Here's how the part is built. I have some questions about the finished solid (model axes, mm). Round coordinates to 2 decimals unless told otherwise and drop trailing zeros. Loops run counter-clockwise (first coordinate to the right, second up) from the corner with the lowest first, then second, coordinate; pieces in that order, holes last. Notation, with made-up numbers: M 53.25,-26.75 L 62.25,-26.75 A24 cw 62.25,-2.75 Z; hole C 18.25,11 d9. An arc over 180 degrees is marked long. Answer as a JSON object with one key per item and string values.
from build123d import *

# Parameters (mm, degrees)
SKETCH1_R           = 88.9
BOSS_EXTRUDE1_DEPTH = 6.35
CUT_EXTRUDE1_REACH  = 8.35
SKETCH2_R           = 1
CUT_EXTRUDE2_REACH  = 8.35
SKETCH4_R           = 1.5875


with BuildPart() as part:
    # Sketch1 → Boss-Extrude1 (new body)
    with BuildSketch(Plane(origin=(0, 0, 0), x_dir=(1, 0, 0), z_dir=(0, 1, 0))):
        Circle(SKETCH1_R)
    extrude(amount=BOSS_EXTRUDE1_DEPTH)

    # Sketch2 → Cut-Extrude1 (cut, up to next)
    with BuildSketch(Plane.XZ, mode=Mode.PRIVATE) as cut_extrude1_sk1:
        with Locations((2.411677935, -76.2)):
            Circle(SKETCH2_R)
    cut_extrude1_tool1 = extrude(cut_extrude1_sk1.sketch, amount=-CUT_EXTRUDE1_REACH, mode=Mode.PRIVATE) & part.part
    add(cut_extrude1_tool1.solids().sort_by_distance((2.411678, 0, -76.2))[0], mode=Mode.SUBTRACT)
    # Sketch2 → Cut-Extrude1 (cut, up to next)
    with BuildSketch(Plane.XZ, mode=Mode.PRIVATE) as cut_extrude1_sk2:
        with Locations((-2.425285476, -76.2)):
            Circle(SKETCH2_R)
    cut_extrude1_tool2 = extrude(cut_extrude1_sk2.sketch, amount=-CUT_EXTRUDE1_REACH, mode=Mode.PRIVATE) & part.part
    add(cut_extrude1_tool2.solids().sort_by_distance((-2.425285, 0, -76.2))[0], mode=Mode.SUBTRACT)
    # Sketch2 → Cut-Extrude1 (cut, up to next)
    with BuildSketch(Plane.XZ, mode=Mode.PRIVATE) as cut_extrude1_sk3:
        with Locations((-76.2, -2.411677935)):
            Circle(SKETCH2_R)
    cut_extrude1_tool3 = extrude(cut_extrude1_sk3.sketch, amount=-CUT_EXTRUDE1_REACH, mode=Mode.PRIVATE) & part.part
    add(cut_extrude1_tool3.solids().sort_by_distance((-76.2, 0, -2.411678))[0], mode=Mode.SUBTRACT)
    # Sketch2 → Cut-Extrude1 (cut, up to next)
    with BuildSketch(Plane.XZ, mode=Mode.PRIVATE) as cut_extrude1_sk4:
        with Locations((-76.2, 2.425285476)):
            Circle(SKETCH2_R)
    cut_extrude1_tool4 = extrude(cut_extrude1_sk4.sketch, amount=-CUT_EXTRUDE1_REACH, mode=Mode.PRIVATE) & part.part
    add(cut_extrude1_tool4.solids().sort_by_distance((-76.2, 0, 2.425285))[0], mode=Mode.SUBTRACT)
    # Sketch2 → Cut-Extrude1 (cut, up to next)
    with BuildSketch(Plane.XZ, mode=Mode.PRIVATE) as cut_extrude1_sk5:
        with Locations((-2.411677935, 76.2)):
            Circle(SKETCH2_R)
    cut_extrude1_tool5 = extrude(cut_extrude1_sk5.sketch, amount=-CUT_EXTRUDE1_REACH, mode=Mode.PRIVATE) & part.part
    add(cut_extrude1_tool5.solids().sort_by_distance((-2.411678, 0, 76.2))[0], mode=Mode.SUBTRACT)
    # Sketch2 → Cut-Extrude1 (cut, up to next)
    with BuildSketch(Plane.XZ, mode=Mode.PRIVATE) as cut_extrude1_sk6:
        with Locations((2.425285476, 76.2)):
            Circle(SKETCH2_R)
    cut_extrude1_tool6 = extrude(cut_extrude1_sk6.sketch, amount=-CUT_EXTRUDE1_REACH, mode=Mode.PRIVATE) & part.part
    add(cut_extrude1_tool6.solids().sort_by_distance((2.425285, 0, 76.2))[0], mode=Mode.SUBTRACT)
    # Sketch2 → Cut-Extrude1 (cut, up to next)
    with BuildSketch(Plane.XZ, mode=Mode.PRIVATE) as cut_extrude1_sk7:
        with Locations((76.2, 2.411677935)):
            Circle(SKETCH2_R)
    cut_extrude1_tool7 = extrude(cut_extrude1_sk7.sketch, amount=-CUT_EXTRUDE1_REACH, mode=Mode.PRIVATE) & part.part
    add(cut_extrude1_tool7.solids().sort_by_distance((76.2, 0, 2.411678))[0], mode=Mode.SUBTRACT)
    # Sketch2 → Cut-Extrude1 (cut, up to next)
    with BuildSketch(Plane.XZ, mode=Mode.PRIVATE) as cut_extrude1_sk8:
        with Locations((76.2, -2.425285476)):
            Circle(SKETCH2_R)
    cut_extrude1_tool8 = extrude(cut_extrude1_sk8.sketch, amount=-CUT_EXTRUDE1_REACH, mode=Mode.PRIVATE) & part.part
    add(cut_extrude1_tool8.solids().sort_by_distance((76.2, 0, -2.425285))[0], mode=Mode.SUBTRACT)

    # Sketch4 → Cut-Extrude2 (cut, up to next)
    with BuildSketch(Plane.XZ, mode=Mode.PRIVATE) as cut_extrude2_sk1:
        with Locations((4.766839139, -13.885779707)):
            Circle(SKETCH4_R)
    cut_extrude2_tool1 = extrude(cut_extrude2_sk1.sketch, amount=-CUT_EXTRUDE2_REACH, mode=Mode.PRIVATE) & part.part
    add(cut_extrude2_tool1.solids().sort_by_distance((4.766839, 0, -13.88578))[0], mode=Mode.SUBTRACT)
    # Sketch4 → Cut-Extrude2 (cut, up to next)
    with BuildSketch(Plane.XZ, mode=Mode.PRIVATE) as cut_extrude2_sk2:
        with Locations((-14.408857547, 2.814686063)):
            Circle(SKETCH4_R)
    cut_extrude2_tool2 = extrude(cut_extrude2_sk2.sketch, amount=-CUT_EXTRUDE2_REACH, mode=Mode.PRIVATE) & part.part
    add(cut_extrude2_tool2.solids().sort_by_distance((-14.408858, 0, 2.814686))[0], mode=Mode.SUBTRACT)
    # Sketch4 → Cut-Extrude2 (cut, up to next)
    with BuildSketch(Plane.XZ, mode=Mode.PRIVATE) as cut_extrude2_sk3:
        with Locations((9.642018407, 11.071093644)):
            Circle(SKETCH4_R)
    cut_extrude2_tool3 = extrude(cut_extrude2_sk3.sketch, amount=-CUT_EXTRUDE2_REACH, mode=Mode.PRIVATE) & part.part
    add(cut_extrude2_tool3.solids().sort_by_distance((9.642018, 0, 11.071094))[0], mode=Mode.SUBTRACT)


solid = part.part
Item 1: I'm going to push flat-ended pins straight in: pin 1 Ø2.5 at (x, z) = (76.2, 2.41) entering from +Y; pin 2 Ø1.2 at (x, z) = (-76.2, -2.41) entering from +Y; pin 3 Ø1 at (y, z) = (4, -67) entering from +X; pin 4 Ø2 at (y, z) = (2.5, 8) entering from +X. Where does each tip first touch, or does it pass through?
Resolved:
{"pin 1": "y = 6.35", "pin 2": "through", "pin 3": "x = 59", "pin 4": "x = 88.62"}
Item 2: I want a section at A-A, the plane y = 1.5. State how many separate pieces and enclosed holes the cut face has, then the cut area to 3 significant figures.
Resolved:
{"separate pieces": "1", "enclosed holes": "11", "area": "24,800 mm²"}
Item 3: Please list where these lines run through material, in increasing order: probe 1 along Z at (x, y) = (2, 4.75); probe 2 along X at (y, z) = (3.5, 75.5); probe 3 along X at (y, z) = (2.75, -76.2). Write a range as from..to.
Resolved:
{"probe 1": "-88.88..-77.11, -75.29..75.29, 77.11..88.88", "probe 2": "-46.94..-3.13, -1.7..1.71, 3.14..46.94", "probe 3": "-45.79..-3.43, -1.43..1.41, 3.41..45.79"}
Item 4: I want a section at C-C, the plane z = 22. Please give me the cut outline in (x, y).
Resolved:
{"outline": "M -86.13,0 L 86.13,0 L 86.13,6.35 L -86.13,6.35 Z"}
Item 5: I want a section at B-B, the plane x = -50. Please give me the cut outline in (y, z), then the cut area to 3 significant figures.
Resolved:
{"outline": "M 0,-73.51 L 6.35,-73.51 L 6.35,73.51 L 0,73.51 Z", "area": "934 mm²"}
